Here's how the part is built. I have some questions about the finished solid (model axes, mm). A direction names the side the tool comes from. Coordinates: 2 decimals unless noted, no trailing zeros. Write each loop counter-clockwise with the first axis right and the second up, starting at its lowest first coordinate (ties: lowest second). Pieces come first, ordered by that corner, then holes. Notation, with made-up numbers: (70.25, -10) -> (111.25, -10) arc R18 ccw to (111.25, 24) -> close; hole circle Ø4 at (28.5, 86). An arc over 180 degrees is marked (long way). Put each result on its own line as item: value. Start each with the question number.
Item 1: If we mould it in two halves opening along Z, with no side actions, what happens to faces 1 (the face through (0, 8.4, 32.2)), 2 (the face through (1.5, -3, 17)), 3 (the face through (0, 0, 35))? For each: released by +Z, released by -Z, zero draft, split by the parting line, or undercut.
Item 2: On a 3-axis mill with a long thin cutter (end or side, diameter ignored), from which of +Z, -Z, +X, -X, +Y, -Y can I reach the whole of each face in a straight line? I mean faces 4 (the face through (0, -30, -1)), 5 (the face through (-1.5, 0, 17)), 6 (the face through (0, -10, 17)). Say none if no direction works.
Item 3: I need wall thicknesses on line 1 (Z direction, x = -10.75, y = -6); line 2 (X direction, y = -8.5, z = 10); line 3 (X direction, y = 7.5, z = 21). Which ranges of each line are inside material? Lowest first, please. Write a range as [from, to].
Item 4: I want a section at D-D, the plane y = 19. List the corners of the cut face in (x, z) for me, then the cut area to 3 significant figures.
Item 5: I want a section at B-B, the plane z = 20.5. List the corners of the cut face in (x, y) for me.
Item 6: For pin 1 (21 mm diameter, centred on y = -2, z = 14, fed in from -X); pin 2 (12 mm diameter, centred on x = -6.5, y = -14, fed in from +Z); pin 3 (0.5 mm diameter, centred on x = 0, z = 34, fed in from +Y), each with a flat end and sliding along its axis, tell me the tip position at first contact or that it passes through.
Item 7: I want a section at C-C, the plane x = 8.25. List the corners of the cut face in (y, z) for me, then the cut area to 3 significant figures.
Item 8: I want a section at A-A, the plane y = -6. List the corners of the cut face in (x, z) for me.
Autodesk Fusion 360 part; units mm, degrees
sketch "Sketch1" plane through (0, 0, 0) normal (0, 0, 1) x (1, 0, 0)
  line L0 (15, 30) -> (-15, 30)
  line L1 (-15, 30) -> (-15, -30)
  line L2 (-15, -30) -> (15, -30)
  line L3 (15, -30) -> (15, 30)
  line L4 (15, 30) -> (-15, -30) construction
  line L5 (-15, 30) -> (15, -30) construction
  line L6 (1.5, 10) -> (-1.5, 10)
  line L7 (-1.5, 10) -> (-1.5, -10)
  line L8 (-1.5, -10) -> (1.5, -10)
  line L9 (1.5, -10) -> (1.5, 10)
  line L10 (1.5, 10) -> (-1.5, -10) construction
  line L11 (-1.5, 10) -> (1.5, -10) construction
  dimension "d1" = 60
  dimension "d2" = 30
  dimension "d3" = 20
  dimension "d4" = 3
extrude "Extrude1" add sketch "Sketch1" against normal blind 3 contours L0 L1 L2 L3 | L6 L7 L8 L9
extrude "Extrude2" add sketch "Sketch1" along normal blind 35 contours L6 L7 L8 L9
sketch "Sketch2" plane through (0, 0, 0) normal (1, 0, 0) x (0, 0, -1)
sketch "Sketch3" plane through (1.5, 0, 0) normal (1, 0, 0) x (0, 0, -1)
  line L0 (0, -10) -> (0, 10)
  line L1 (0, 10) -> (-35, 10)
  line L2 (-35, 10) -> (-35, -10)
  line L3 (-35, -10) -> (0, -10)
  line L4 (0, 10) -> (-33, 10)
  line L5 (-33, 10) -> (-33, 8) construction
  line L6 (-33, 8) -> (0, 8)
  line L7 (0, 8) -> (0, 10)
  arc A0 (-33, 10) -> (-31, 8) centre (-31, 10) ccw
  dimension "d9" = 2
  dimension "d10" = 33
  dimension "d15" = 4
extrude "Extrude3" cut sketch "Sketch3" against normal through all contours L0 L1 L4 L6 L7 A0
fillet "Fillet4" radius 1 2 edges at (1.5, 8, 15.5) (1.5, 8.5858, 32.4142)
fillet "Fillet5" radius 1 2 edges at (-1.5, 8.5858, 32.4142) (-1.5, 8, 15.5)
fillet "Fillet6" radius 1 5 edges at (-1.5, 10, 34.5) (-1.2071, 10, 33.2929) (0, 10, 33) (1.2071, 10, 33.2929) (1.5, 10, 34.5)
Calculated:
1. face 1: undercut
1. face 2: zero draft
1. face 3: released by +Z
2. face 4: +Z, -Z, +X, -X, -Y
2. face 5: +Z, -X, +Y, -Y
2. face 6: +Z, +X, -X, -Y
3. line 1: z = [-3, 0]
3. line 2: x = [-1.5, 1.5]
3. line 3: x = [-1.37, 1.37]
4. outline: (-15, -3) -> (15, -3) -> (15, 0) -> (-15, 0) -> close
4. area: 90.0 mm2
5. outline: (-1.5, -10) -> (1.5, -10) -> (1.5, 7) arc R1 ccw to (0.5, 8) -> (-0.5, 8) arc R1 ccw to (-1.5, 7) -> close
6. pin 1: stops at x = -1.5
6. pin 2: stops at z = 0
6. pin 3: stops at y = 10
7. outline: (-30, -3) -> (30, -3) -> (30, 0) -> (-30, 0) -> close
7. area: 180 mm2
8. outline: (-15, -3) -> (15, -3) -> (15, 0) -> (1.5, 0) -> (1.5, 35) -> (-1.5, 35) -> (-1.5, 0) -> (-15, 0) -> close
